Verification items for the finished model (mm, model axes). Face numbers are marked on the shaded views. A direction names the side the tool comes from. Give positions to 0.01 mm unless a question says otherwise; leave off trailing zeros. Answer in a Markdown table with one row per item.
```python
from build123d import *

# Parameters (mm, degrees)
BOSS_EXTRUDE1_DEPTH     = 55
SKETCH2_R               = 1.5000000000000007
CUT_EXTRUDE1_DEPTH      = 2.8
CUT_EXTRUDE2_START      = -2.8
SKETCH3_R               = 1.5000000000000007
CUT_EXTRUDE2_DEPTH      = 2.8
CUT_EXTRUDE3_DEPTH      = 5
CUT_EXTRUDE3_DEPTH_BACK = 1
CUT_EXTRUDE4_DEPTH      = 1
CUT_EXTRUDE4_DEPTH_BACK = 1
FILLET1_R               = 2
FILLET2_R               = 1


with BuildPart() as part:
    # Sketch1 → Boss-Extrude1 (new body)
    with BuildSketch(Plane(origin=(0, 0, 0), x_dir=(1, 0, 0), z_dir=(0, 1, 0))):
        with BuildLine():
            Line((-18.500000000000032, 1.9999999999999996), (-21.500000000000068, 1.9999999999999996))
            ThreePointArc((-21.500000000000053, 1.9999999999999463), (-22.499999999999986, -1.91e-15), (-21.50000000000005, -1.9999999999999476))
            Line((-21.500000000000064, -2.0000000000000004), (-18.500000000000036, -2.0000000000000004))
            ThreePointArc((-18.50000000000003, -2.0000000000000226), (-17.763932022500214, -1.1180339887499129), (-17.499999999999993, -6.1e-16))
            ThreePointArc((-17.499999999999993, 0), (-17.763932022500214, 1.1180339887499113), (-18.500000000000025, 2.0000000000000213))
        make_face()
        with BuildLine():
            ThreePointArc((-18.500000000000025, 2.000000000000021), (-20.00000000000005, 2.4999999999999947), (-21.500000000000053, 1.9999999999999463))
            Line((-21.500000000000068, 1.9999999999999996), (-18.500000000000032, 1.9999999999999996))
        make_face()
        with BuildLine():
            Line((-18.500000000000036, -2.0000000000000004), (-21.500000000000064, -2.0000000000000004))
            ThreePointArc((-21.50000000000005, -1.9999999999999476), (-20.000000000000053, -2.4999999999999947), (-18.50000000000003, -2.0000000000000226))
        make_face()
        with BuildLine():
            Line((-21.500000000000068, 1.9999999999999996), (-27.49999999999999, 1.9999999999999996))
            Line((-27.49999999999999, 1.9999999999999996), (-27.49999999999999, -2.0000000000000004))
            Line((-27.49999999999999, -2.0000000000000004), (-21.500000000000064, -2.0000000000000004))
            ThreePointArc((-21.50000000000005, -1.9999999999999476), (-22.499999999999986, -1.91e-15), (-21.500000000000053, 1.9999999999999463))
        make_face()
        with BuildLine():
            Line((18.49999999999991, 1.9999999999999996), (-18.500000000000032, 1.9999999999999996))
            ThreePointArc((-18.500000000000025, 2.0000000000000213), (-17.763932022500214, 1.1180339887499113), (-17.499999999999993, 0))
            ThreePointArc((-17.499999999999993, -6.1e-16), (-17.763932022500214, -1.1180339887499129), (-18.50000000000003, -2.0000000000000226))
            Line((-18.500000000000036, -2.0000000000000004), (18.499999999999925, -2.0000000000000004))
            ThreePointArc((18.499999999999932, -1.9999999999999478), (17.5, -1.91e-15), (18.49999999999993, 1.9999999999999456))
        make_face()
        with BuildLine():
            ThreePointArc((21.49999999999997, 2.00000000000002), (19.99999999999994, 2.4999999999999982), (18.49999999999993, 1.9999999999999456))
            Line((18.49999999999991, 1.9999999999999996), (21.499999999999968, 1.9999999999999996))
        make_face()
        with BuildLine():
            Line((21.499999999999968, 1.9999999999999996), (18.49999999999991, 1.9999999999999996))
            ThreePointArc((18.49999999999993, 1.9999999999999456), (17.5, -1.91e-15), (18.499999999999932, -1.9999999999999478))
            Line((18.49999999999992, -2.0000000000000004), (21.499999999999954, -2.0000000000000004))
            ThreePointArc((21.499999999999964, -2.0000000000000244), (22.23606797749978, -1.1180339887499124), (22.5, -6.1e-16))
            ThreePointArc((22.5, 0), (22.23606797749978, 1.11803398874991), (21.49999999999997, 2.00000000000002))
        make_face()
        with BuildLine():
            Line((21.499999999999954, -2.0000000000000004), (18.49999999999992, -2.0000000000000004))
            ThreePointArc((18.499999999999932, -1.9999999999999478), (19.999999999999936, -2.4999999999999982), (21.499999999999964, -2.0000000000000244))
        make_face()
        with BuildLine():
            Line((27.50000000000001, 1.9999999999999996), (21.499999999999968, 1.9999999999999996))
            ThreePointArc((21.49999999999997, 2.00000000000002), (22.23606797749978, 1.11803398874991), (22.5, 0))
            ThreePointArc((22.5, -6.1e-16), (22.23606797749978, -1.1180339887499124), (21.499999999999964, -2.0000000000000244))
            Line((21.499999999999954, -2.0000000000000004), (27.50000000000001, -2.0000000000000004))
            Line((27.50000000000001, -2.0000000000000004), (27.50000000000001, 1.9999999999999996))
        make_face()
    extrude(amount=BOSS_EXTRUDE1_DEPTH)

    # Sketch2 → Cut-Extrude1 (cut)
    with BuildSketch(Plane(origin=(0, 55, 0), x_dir=(1, 0, 0), z_dir=(0, 1, 0))):
        with Locations(Location((-19.99999999999999, 0, 0), (0, 0, 270))):
            Circle(SKETCH2_R)
        with Locations(Location((20, 0, 0), (0, 0, 270))):
            Circle(SKETCH2_R)
    extrude(amount=-CUT_EXTRUDE1_DEPTH, mode=Mode.SUBTRACT)

    # Sketch3 → Cut-Extrude2 (cut)
    with BuildSketch(Plane.XZ.offset(CUT_EXTRUDE2_START)):
        with Locations(Location((-19.99999999999999, 0, 0), (0, 0, 90))):
            Circle(SKETCH3_R)
        with Locations(Location((20, 0, 0), (0, 0, 90))):
            Circle(SKETCH3_R)
    extrude(amount=CUT_EXTRUDE2_DEPTH, mode=Mode.SUBTRACT)

    # Sketch4 → Cut-Extrude3 (cut, two sides: drawn at the far end of the back side and taken through both)
    with BuildSketch(Plane.XY.offset(2.0000000000000004).offset(-CUT_EXTRUDE3_DEPTH_BACK)):
        Polygon((-27.500000000000018, 50), (27.500000000000007, 50), (27.50000000000001, 5.000000000000008), (-27.50000000000001, 5.000000000000008), align=None)
    extrude(amount=CUT_EXTRUDE3_DEPTH + CUT_EXTRUDE3_DEPTH_BACK, mode=Mode.SUBTRACT)

    # Sketch5 → Cut-Extrude4 (cut, two sides: drawn at the far end of the back side and taken through both)
    with BuildSketch(Plane(origin=(0, 0, -1.9999999999999996), x_dir=(-1, 0, 0), z_dir=(0, 0, -1)).offset(-CUT_EXTRUDE4_DEPTH_BACK)):
        Polygon((-27.49999999999999, 50), (27.49999999999999, 50), (27.499999999999986, 5.000000000000001), (-27.49999999999998, 5.000000000000001), align=None)
    extrude(amount=CUT_EXTRUDE4_DEPTH + CUT_EXTRUDE4_DEPTH_BACK, mode=Mode.SUBTRACT)

    # Fillet1
    fillet1_edges = [part.edges().sort_by_distance(p)[0] for p in [
        (-27.49999999999999, 52.5, 2.0000000000000004),
    ]]
    fillet(fillet1_edges, radius=FILLET1_R)
    fillet1_2_edges = [part.edges().sort_by_distance(p)[0] for p in [
        (-27.49999999999999, 2.5000000000000004, -1.9999999999999996),
    ]]
    fillet(fillet1_2_edges, radius=FILLET1_R - 0.0004)  # a hair under: the kernel refuses the full size
    fillet1_3_edges = [part.edges().sort_by_distance(p)[0] for p in [
        (27.50000000000001, 52.5, 2.0000000000000004),
    ]]
    fillet(fillet1_3_edges, radius=FILLET1_R)
    fillet1_4_edges = [part.edges().sort_by_distance(p)[0] for p in [
        (27.50000000000001, 2.5000000000000004, -1.9999999999999996),
    ]]
    fillet(fillet1_4_edges, radius=FILLET1_R - 0.0004)  # a hair under: the kernel refuses the full size

    # Fillet2
    fillet2_edges = [part.edges().sort_by_distance(p)[0] for p in [
        (-19.999999999999986, 50, -2.499999999999992),
        (19.999999999999996, 50, -2.500000000000009),
        (19.999999999999996, 5.000000000000001, -2.500000000000009),
        (-19.999999999999986, 5.000000000000001, -2.499999999999992),
        (-5.684e-14, 50, -1.9999999999999996),
        (23.500199999999992, 5.000000000000001, -1.9999999999999996),
        (-5.151e-14, 5.000000000000001, -1.9999999999999996),
        (23.500200169244646, 50, -1.9999999999999996),
        (-26.5002999949995, 50, -1.7320466614179624),
        (26.50030014156478, 50, -1.7320465767871778),
        (-23.500200000000024, 5.000000000000001, -1.9999999999999996),
        (-26.50029999499948, 5.000000000000001, -1.7320466614179733),
        (26.500299994999555, 5.000000000000001, -1.732046661417944),
        (-23.500000000000025, 5.000000000000008, 2.0000000000000004),
        (-26.49999999999999, 5.000000000000007, 1.7320508075688776),
        (26.500000103238282, 5.000000000000007, 1.7320507479642298),
        (23.499999999999982, 50, 2.0000000000000004),
        (-26.499999999999982, 50, 1.7320508075688823),
        (26.50000000000001, 50, 1.732050807568878),
        (-20.000000000000053, 50, 2.4999999999999925),
        (-23.50000000000002, 50, 2.0000000000000004),
        (19.999999999999932, 50, 2.499999999999999),
        (-5.329e-14, 50, 2.0000000000000004),
        (-20.000000000000053, 5.000000000000008, 2.4999999999999925),
        (-5.507e-14, 5.000000000000008, 2.0000000000000004),
        (19.999999999999932, 5.000000000000008, 2.499999999999999),
        (23.500000119209272, 5.000000000000008, 2.0000000000000004),
        (-23.500200000000024, 50, -1.9999999999999996),
    ]]
    fillet(fillet2_edges, radius=FILLET2_R - 0.0001)  # a hair under: the kernel refuses the full size


solid = part.part
```
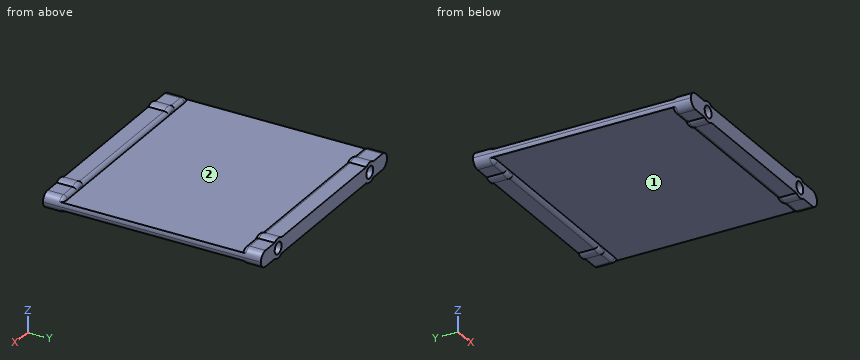
Item 1: Go/stop test with flat-tipped pins: pin 1 (4.5 mm diameter, centred on x = 23.5, y = 2.5, fed in from +Z); pin 2 (12 mm diameter, centred on x = -13.5, y = 15, fed in from -Z); pin 3 (4.5 mm diameter, centred on x = 23, y = 1.5, fed in from -Z). Record where each tip stops, or that it passes through.
Reported:
| item | result |
|---|---|
| pin 1 | stops at z = 2.17 |
| pin 2 | stops at z = -1 |
| pin 3 | stops at z = -2.38 |
Item 2: Scan lines: L1, parallel to Z at x = 20, y = 0.8; L2, parallel to Z at x = 9, y = 25; L3, parallel to Z at x = 16.5, y = 53.5. Record each from-to range of solid material in increasing order. Write a range as [from, to].
Reported:
| item | result |
|---|---|
| L1 | z = [-2.5, -1.5], [1.5, 2.5] |
| L2 | z = [-1, 1] |
| L3 | z = [-2, 2] |
Item 3: Tool access check on the marked faces 1 and 2. Record the directions out of +Z, -Z, +X, -X, +Y, -Y that give a thin tool (end or side, any length) a straight path to the whole face; none if there is none.
Reported:
| item | result |
|---|---|
| face 1 | -Z, +X, -X |
| face 2 | +Z, +X, -X |
